Could you check a few things on this drawing? It's one solid part, dimensions in mm from its lowest x, y, z. A direction names the side the tool comes from. Give positions to 0.01 mm unless a question says otherwise; leave off trailing zeros. Order: outer loops, then holes, each group sorted by start corner. A loop starts at its lowest first (then second) coordinate and runs counter-clockwise, first axis right, second up.
(1) Imagine slicing it at C-C, the plane x = 39. Write out the boundary of the cut face in (y, z), then the cut area to 3 significant figures.
(2) Will these pins go through, and if not, where does the flat tip stop? pin 1 (1.8 mm diameter, centred on x = 39, y = 8.5, fed in from -Z); pin 2 (2.5 mm diameter, centred on y = 12, z = 5, fed in from -X); pin 3 (1.6 mm diameter, centred on x = 8.5, z = 1, fed in from -Y); pin 4 (1 mm diameter, centred on y = 21.5, z = 1, fed in from -X).
(3) Imagine slicing it at B-B, the plane z = 7.75. Write out the boundary of the cut face in (x, y).
(4) Imagine slicing it at A-A, the plane y = 13. Write out the boundary of the cut face in (x, z), then the cut area to 3 significant figures.
(5) If I drill on probe 1 along X at (y, z) = (10, 8.45); probe 2 along Y at (x, z) = (2.5, 1.05); probe 3 along Y at (x, z) = (39, 8), over which ranges is the centre line in solid material (lowest first)?
(6) Imagine slicing it at D-D, the plane y = 10. Write out the boundary of the cut face in (x, z), then the cut area to 4 significant figures.
(7) On a 3-axis mill with a long thin cutter (end or side, diameter ignored), from which of +Z, -Z, +X, -X, +Y, -Y can I reach the whole of each face in a straight line? I mean the marked faces 1, 2 and 3. Say none if no direction works.
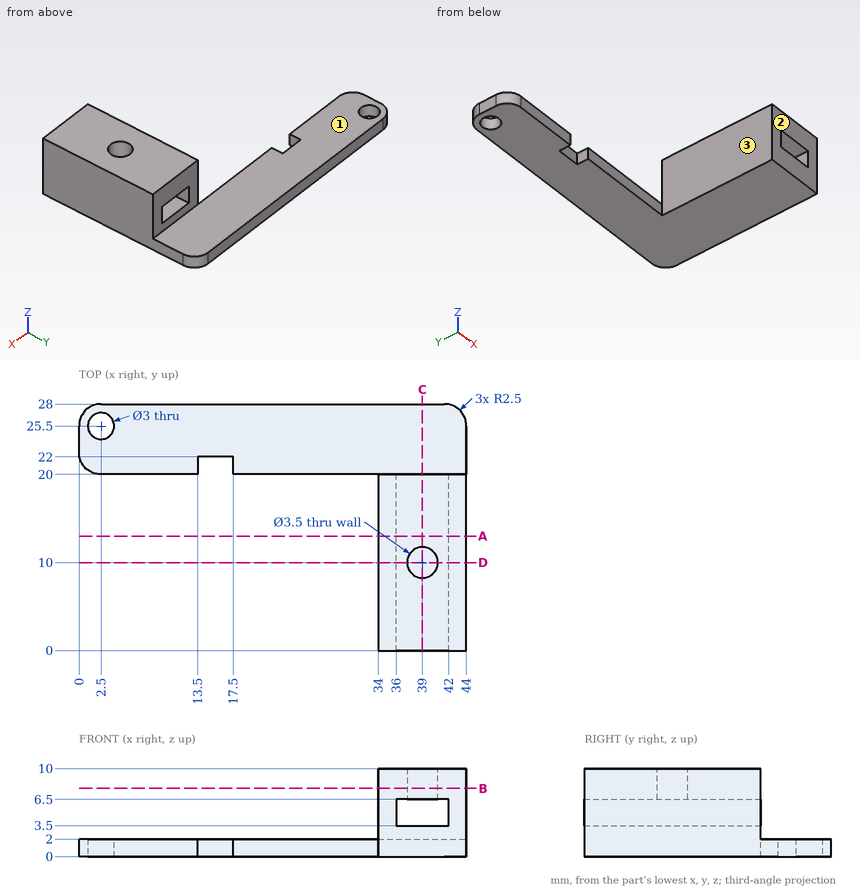
Answer block:
1. outline: (0, 0) - (28, 0) - (28, 2) - (20, 2) - (20, 3.5) - (0, 3.5) - close; (0, 6.5) - (8.25, 6.5) - (8.25, 10) - (0, 10) - close; (11.75, 6.5) - (20, 6.5) - (20, 10) - (11.75, 10) - close
1. area: 144 mm2
2. pin 1: stops at z = 0
2. pin 2: stops at x = 34
2. pin 3: stops at y = 20
2. pin 4: stops at x = 0.05
3. outline: (34, 0) - (44, 0) - (44, 20) - (34, 20) - close; hole circle Ø3.5 at (39, 10)
4. outline: (34, 0) - (44, 0) - (44, 10) - (34, 10) - close; hole (36, 3.5) - (42, 3.5) - (42, 6.5) - (36, 6.5) - close
4. area: 82.0 mm2
5. probe 1: x = 34 to 37.25, 40.75 to 44
5. probe 2: y = 20 to 24, 27 to 28
5. probe 3: y = 0 to 8.25, 11.75 to 20
6. outline: (34, 0) - (44, 0) - (44, 10) - (40.75, 10) - (40.75, 6.5) - (42, 6.5) - (42, 3.5) - (36, 3.5) - (36, 6.5) - (37.25, 6.5) - (37.25, 10) - (34, 10) - close
6. area: 69.75 mm2
7. face 1: +Z, +X, -X, +Y
7. face 2: +Z, -Z, +X, -X, -Y
7. face 3: +Z, -Z, -X, -Y
